Could you check a few things on this model? Use its own coordinates, in mm. Face numbers are marked on the shaded views. A direction names the side the tool comes from. Round coordinates to 2 decimals unless told otherwise and drop trailing zeros. Loops run counter-clockwise (first coordinate to the right, second up) from the corner with the lowest first, then second, coordinate; pieces in that order, holes last. Notation, with made-up numbers: (-14, -2) - (0, -2) arc R15 ccw to (0, 22) - close; hole circle Ø11 at (41, 11). An arc over 180 degrees is marked (long way). Answer as CSV lines item,"result". Start each with the question number.
1) Suppose I cut it at A-A, the plane x = 12. Write out the boundary of the cut face in (y, z).
2) Please list where these lines run through material, in increasing order: line 1 along X through (y, z) = (-2.5, -1.25); line 2 along X through (y, z) = (-0.25, 1); line 3 along Y through (x, z) = (10, -1.75).
3) We'd pull the mould along Y, two halves only. Please class the marked faces 1, 2 and 3: pulls with the +Y half, pulls with the -Y half, needs draft (parallel to the pull), parting line crosses it, or undercut.
4) Which directions (+Z, -Z, +X, -X, +Y, -Y) give clear straight access to the entire face, cutting with the end or side of a thin tool? Please do the marked faces 4, 5 and 6.
5) I'm going to push flat-ended pins straight in: pin 1 Ø0.6 at (y, z) = (-1.5, -0.5) entering from -X; pin 2 Ø1.5 at (x, y) = (7, 0.5) entering from +Z; pin 3 Ø0.7 at (y, z) = (0.5, 1) entering from -X; pin 4 Ø1.5 at (x, y) = (8.5, 1.5) entering from -Z. Where does each tip first touch, or does it pass through?
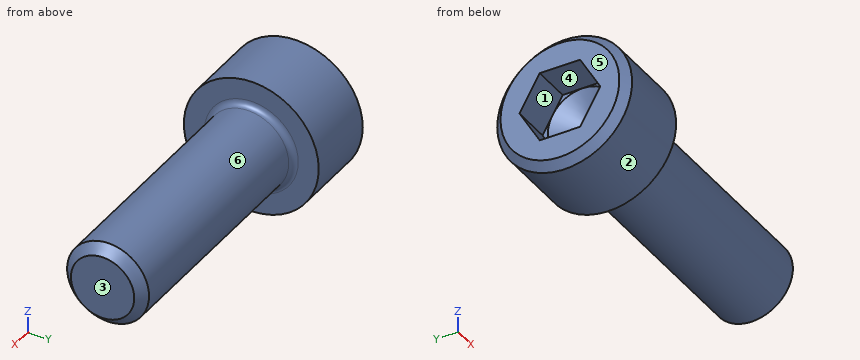
```python
from build123d import *

# Parameters (mm, degrees)
FILLET1_R   = 0.3048
HEX_2_DEPTH = 1.9558


with BuildPart() as part:
    # BodySke → Base-Revolve (revolve)
    with BuildSketch(Plane.XY):
        Polygon((0, 0), (0, 3.0226), (0.4064, 3.429), (4.1656, 3.429), (4.1656, 2.0828), (16.39316, 2.0828), (16.8656, 1.61036), (16.8656, 0), align=None)
    revolve(axis=Axis((-31.75, 0, 0), (1, 0, 0)))

    # Fillet1
    fillet1_edges = [part.edges().sort_by_distance(p)[0] for p in [
        (4.1656, -2.0828, 0),
    ]]
    fillet(fillet1_edges, radius=FILLET1_R)

    # Sketch2 → Hex-PreBroach (revolve, cut)
    with BuildSketch(Plane.XY):
        Polygon((0, 1.778), (1.9558, 1.778), (2.982328779, 0), (0, 0), align=None)
    revolve(axis=Axis((0, 0, 0), (1, 0, 0)), mode=Mode.SUBTRACT)

    # Sketch3 → Hex 2 (cut)
    with BuildSketch(Plane(origin=(0, 0, 0), x_dir=(0, 0.5, 0.866025404), z_dir=(-1, 0, 0))):
        Polygon((1.026528779, 1.778), (-1.026528779, 1.778), (-2.053057557, 0), (-1.026528779, -1.778), (1.026528779, -1.778), (2.053057557, 0), align=None)
    extrude(amount=-HEX_2_DEPTH, mode=Mode.SUBTRACT)


solid = part.part
```
Filled sheet:
1,outline,"circle Ø4.17 at (0, 0)"
2,line 1,"0 to 4.17"
2,line 2,"2.39 to 16.87"
2,line 3,"-1.13 to 1.13"
3,face 1,"undercut"
3,face 2,"parting line crosses it"
3,face 3,"needs draft"
4,face 4,"-X"
4,face 5,"+Z, -Z, -X, +Y, -Y"
4,face 6,"+X"
5,pin 1,"x = 0"
5,pin 2,"z = 2.08"
5,pin 3,"x = 2.13"
5,pin 4,"z = -1.94"
